For this review, take the finished solid that the model builds, in its own axes (mm). Face numbers are marked on the shaded views. Give positions to 0.01 mm unless a question says otherwise; leave off trailing zeros. Loops run counter-clockwise (first coordinate to the right, second up) from the corner with the lowest first, then second, coordinate; pieces in that order, holes last. Notation, with made-up numbers: (-23, 35) - (33, 35) arc R35 cw to (33, 67) - close; hole circle Ø1 at (47, 16). An arc over 180 degrees is marked (long way). Put each result on its own line as item: value.
from build123d import *

# Parameters (mm, degrees)
F0_W      = 42
F0_H      = 60
F1_DEPTH  = 25
F2_R      = 5.1
F3_DEPTH  = 25.001
F1_FACE_W = 42
F1_FACE_H = 60
F1_FACE_R = 5.1
F4_DEPTH  = 25
F5_R      = 8.75
F6_DEPTH  = 30
F7_R      = 5.1
F8_DEPTH  = 60


with BuildPart() as f1:
    # F0 (on Top) → F1 (new body)
    with BuildSketch(Plane.XY):
        with Locations((-30.522955, 4.610215)):
            Rectangle(F0_W, F0_H)
    extrude(amount=F1_DEPTH)

    # F2 (on face) → F3 (cut, through all)
    with BuildSketch(Plane.XY.offset(25)):
        with Locations((-21.522955, 22.610215)):
            Circle(F2_R)
    extrude(amount=-F3_DEPTH, mode=Mode.SUBTRACT)

    # F1_face (on face) → F4 (join)
    with BuildSketch(Plane(origin=(-30.522955, 4.610215, 25), x_dir=(1, 0, 0), z_dir=(0, 0, 1))):
        Rectangle(F1_FACE_W, F1_FACE_H)
        with Locations((9, 18)):
            Circle(F1_FACE_R, mode=Mode.SUBTRACT)
    extrude(amount=F4_DEPTH)

    # F5 (on face) → F6 (cut)
    with BuildSketch(Plane.XZ.offset(25.389785)):
        with Locations((-39.522955, 38)):
            Circle(F5_R)
    extrude(amount=-F6_DEPTH, mode=Mode.SUBTRACT)

    # F7 (on face) → F8 (cut)
    with BuildSketch(Plane.XZ.offset(-4.610215)):
        with Locations((-39.522955, 38)):
            Circle(F7_R)
    extrude(amount=-F8_DEPTH, mode=Mode.SUBTRACT)


solid = f1.part
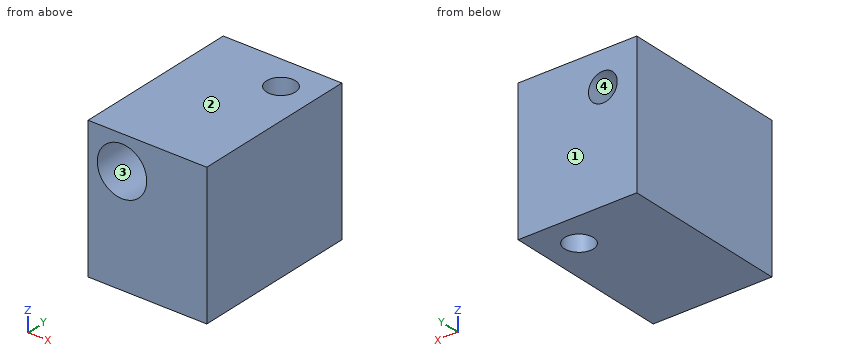
1) Take a section at D-D on z = 26. State the section outline as (x, y) points.
Geometry check:
outline: (-51.52, -25.39) - (-9.52, -25.39) - (-9.52, 34.61) - (-51.52, 34.61) - close; hole circle Ø10.2 at (-21.52, 22.61)
2) Take a section at C-C on x = -32.5. State the section outline as (y, z) points, and give its area (3 significant figures).
Geometry check:
outline: (-25.39, 0) - (34.61, 0) - (34.61, 50) - (-25.39, 50) - (-25.39, 43.22) - (4.61, 43.22) - (4.61, 32.78) - (-25.39, 32.78) - close
area: 2,690 mm²
3) Insertion check: pin 1 Ø6 at (x, y) = (-21.52, 22.61) entering from -Z; pin 2 Ø14 at (x, z) = (-40.5, 38) entering from -Y. Each pin has a flat end and moves straight along its axis. Give the tip position at first contact, or say it passes through.
Geometry check:
pin 1: passes through
pin 2: stops at y = 4.61
4) Take a section at B-B on y = 0. State the section outline as (x, z) points.
Geometry check:
outline: (-51.52, 0) - (-9.52, 0) - (-9.52, 50) - (-51.52, 50) - close; hole circle Ø17.5 at (-39.52, 38)
5) Take a section at A-A on z = 38. State the section outline as (x, y) points.
Geometry check:
outline: (-51.52, -25.39) - (-48.27, -25.39) - (-48.27, 4.61) - (-44.62, 4.61) - (-44.62, 34.61) - (-51.52, 34.61) - close; (-34.42, 4.61) - (-30.77, 4.61) - (-30.77, -25.39) - (-9.52, -25.39) - (-9.52, 34.61) - (-34.42, 34.61) - close; hole circle Ø10.2 at (-21.52, 22.61)
6) Wall thickness on line 1 (Y direction, x = -47, z = 37); line 2 (X direction, y = 18, z = 15.5); line 3 (Z direction, x = -36, y = 23): over which ranges is each line inside the solid? List them lowest first.
Geometry check:
line 1: y = 4.61 to 34.61
line 2: x = -51.52 to -23.7, -19.34 to -9.52
line 3: z = 0 to 34.31, 41.69 to 50
7) Draft analysis for pull direction Z (two halves, no side actions). For the marked faces 1, 2, 3 and 4, state which applies: pulls with the +Z half, pulls with the -Z half, needs draft (parallel to the pull), parting line crosses it, or undercut.
Geometry check:
face 1: needs draft
face 2: pulls with the +Z half
face 3: undercut
face 4: undercut
